For this review, take the finished solid that the model builds, in its own axes (mm). Round coordinates to 2 decimals unless told otherwise and drop trailing zeros. Loops run counter-clockwise (first coordinate to the right, second up) from the corner with the lowest first, then second, coordinate; pieces in that order, holes last. Notation, with made-up numbers: M -30,52 L 6,52 A19 ccw 6,85 Z; hole C 10,64 d11. An arc over 180 degrees is marked long. One line per question, with ' | ' between items. Start each with the question number.
1) We need section A-A (z = -4). Give the boundary of the cut face in (x, y).
2) For pin 1 Ø1 at (x, y) = (1.5, 9) entering from -Z, flat-tipped, find the tip position at first contact; note if it passes through.
3) For probe 1 along Z at (x, y) = (8.25, 4.5); probe 2 along X at (y, z) = (1.25, -15.5); probe 3 along Z at (x, y) = (9.25, 1.25), list the stretches that pass through material, from the lowest coordinate up. Write a range as from..to.
Autodesk Inventor part; units mm, degrees
ref_plane "YZ Plane" through (0, 0, 0) normal (1, 0, 0) x (0, 1, 0)
ref_plane "XZ Plane" through (0, 0, 0) normal (0, 1, 0) x (-1, 0, 0)
ref_plane "XY Plane" through (0, 0, 0) normal (0, 0, 1) x (1, 0, 0)
sketch "草图1" plane through (0, 0, 0) normal (0, 1, 0) x (-1, 0, 0)
  line L0 (10, 25) -> (-10, 25)
  line L1 (-10, 25) -> (-10, -25)
  line L2 (-10, -25) -> (10, -25)
  line L3 (10, -25) -> (10, 25)
  point P0 (0, 0)
  dimension "d0" = 20
  dimension "d1" = 50
extrude "拉伸1" add sketch "草图1" along normal blind 10
fillet "圆角1" radius 2 12 edges at (-10, 5, -25) (-10, 5, 25) (-10, 0, 0) (-10, 10, 0) (10, 5, -25) (0, 0, -25) (0, 10, -25) (10, 5, 25) (10, 0, 0) (10, 10, 0) (0, 0, 25) (0, 10, 25)
properties part number "升降板"
Answers below:
1) outline: M -10,2 A2 ccw -8,0 L 8,0 A2 ccw 10,2 L 10,8 A2 ccw 8,10 L -8,10 A2 ccw -10,8 Z
2) pin 1: z = -24.94
3) probe 1: -24.98..24.98 | probe 2: -9.85..9.85 | probe 3: -24.37..24.37
